Build history of the part. All positions in model axes, mm. A direction names the side the tool comes from. Round coordinates to 2 decimals unless told otherwise and drop trailing zeros. Write each loop counter-clockwise with the first axis right and the second up, starting at its lowest first coordinate (ties: lowest second). Pieces come first, ordered by that corner, then holes. Notation, with made-up numbers: (6.5, -18.5) -> (18.5, -18.5) arc R22 cw to (18.5, 0.5) -> close; hole circle Ø11 at (47, 59). An arc over 180 degrees is marked (long way). Answer in a Markdown table with one row per item. Add a question column.
from build123d import *

# Parameters (mm, degrees)
F0_W     = 38.1
F0_H     = 25.4
F1_DEPTH = 50.8
F3_DEPTH = 12.7


with BuildPart() as f1:
    # F0 (on Right) → F1 (new body)
    with BuildSketch(Plane.YZ):
        with Locations((19.05, 12.7)):
            Rectangle(F0_W, F0_H)
    extrude(amount=F1_DEPTH)

    # F2 (on face) → F3 (cut)
    with BuildSketch(Plane.XY.offset(25.4)):
        Polygon((0, 12.404651), (16.126048, 0), (50.8, 0), (50.8, 19.05), (0, 31.631861), align=None)
    extrude(amount=-F3_DEPTH, mode=Mode.SUBTRACT)


solid = f1.part
(1) Mould opens along Y. For faces 4 (the face through (25.76, 25.25, 19.14)), 5 (the face through (25, 38.1, 13)), 6 (the face through (19, 0, 10)) say: pulls with the +Y half, pulls with the -Y half, needs draft (parallel to the pull), parting line crosses it, or undercut.
(2) Drop a flat-ended pin along its axis: P1, Ø6, axis at x = 31, y = 11, coming from the +Z side. Give the stop position or say it passes through.
(3) Saw through at C-C (y = 21). List the corners of the cut face in (x, z), plus the area to 3 significant figures.
(4) Which spindle directions (+Z, -Z, +X, -X, +Y, -Y) get a long thin tool onto all of the face, cutting with end or side? Do faces 1 (the face through (25, 13, 12.7)), 2 (the face through (31, 31, 25.4)), 3 (the face through (7.95, 6.29, 19.14)). Say none if no direction does.
(5) Saw through at A-A (z = 19). List the corners of the cut face in (x, y), plus the area to 3 significant figures.
(6) Probe line 1 along Z through (x, y) = (31, 22); line 2 along Y through (x, z) = (47, 15.5); line 3 along Y through (x, z) = (33, 16.25). List the from-to ranges inside material, lowest first.
(7) Saw through at B-B (x = 14). List the corners of the cut face in (y, z).
(8) Saw through at D-D (x = 23). List the corners of the cut face in (y, z), plus the area to 3 significant figures.
Answer sheet:
| question | item | result |
|---|---|---|
| 1 | face 4 | undercut |
| 1 | face 5 | pulls with the +Y half |
| 1 | face 6 | pulls with the -Y half |
| 2 | P1 | stops at z = 12.7 |
| 3 | outline | (0, 0) -> (50.8, 0) -> (50.8, 25.4) -> (42.93, 25.4) -> (42.93, 12.7) -> (0, 12.7) -> close |
| 3 | area | 745 mm² |
| 4 | face 1 | +Z |
| 4 | face 2 | +Z, +X, -X, +Y, -Y |
| 4 | face 3 | +Z, +X |
| 5 | outline | (0, 0) -> (16.13, 0) -> (0, 12.4) -> close; (0, 31.63) -> (50.8, 19.05) -> (50.8, 38.1) -> (0, 38.1) -> close |
| 5 | area | 748 mm² |
| 6 | line 1 | z = 0 to 12.7 |
| 6 | line 2 | y = 19.99 to 38.1 |
| 6 | line 3 | y = 23.46 to 38.1 |
| 7 | outline | (0, 0) -> (38.1, 0) -> (38.1, 25.4) -> (28.16, 25.4) -> (28.16, 12.7) -> (1.64, 12.7) -> (1.64, 25.4) -> (0, 25.4) -> close |
| 8 | outline | (0, 0) -> (38.1, 0) -> (38.1, 25.4) -> (25.94, 25.4) -> (25.94, 12.7) -> (0, 12.7) -> close |
| 8 | area | 638 mm² |
